Part print with two shaded views. Sizes in mm from the minimum x, y, z corner. A direction names the side the tool comes from. Round coordinates to 2 decimals unless told otherwise and drop trailing zeros. Write each loop counter-clockwise with the first axis right and the second up, starting at its lowest first coordinate (ties: lowest second). Pieces come first, ordered by that corner, then holes. Notation, with made-up numbers: (34, -24.75) -> (72, -24.75) arc R26 cw to (72, 9.25) -> close; hole circle Ø8 at (-4, -1.5). An arc over 180 degrees is marked (long way). Put each result on its own line as item: value. Start each with the question number.
1. Saw through at A-A on y = 8.5. List the corners of the cut face in (x, z) (1 decimal).
2. 3-axis set-ups, long thin cutter, end or side, ignore diameter. For the marked faces 1 and 2: which of +Z, -Z, +X, -X, +Y, -Y reach the whole face in a straight line?
3. Flat gauge pins, fed straight in: P1, Ø2, axis at x = 29, y = 8.5, coming from the +Z side; P2, Ø12, axis at x = 14, z = 8.5, coming from the -Y side; P3, Ø1.9, axis at y = 10, z = 15.5, coming from the +X side. Where does each tip first touch, or does it go through?
4. Saw through at B-B on z = 7.5. List the corners of the cut face in (x, y).
5. Drill centre lines: line 1 (Z direction, x = 5.08, y = 9.75) (1 decimal); line 2 (X direction, y = 8, z = 17.78) (1 decimal); line 3 (Y direction, x = 2.5, z = 21.5). Where is each one in solid material? Low to high. Write a range as from..to.
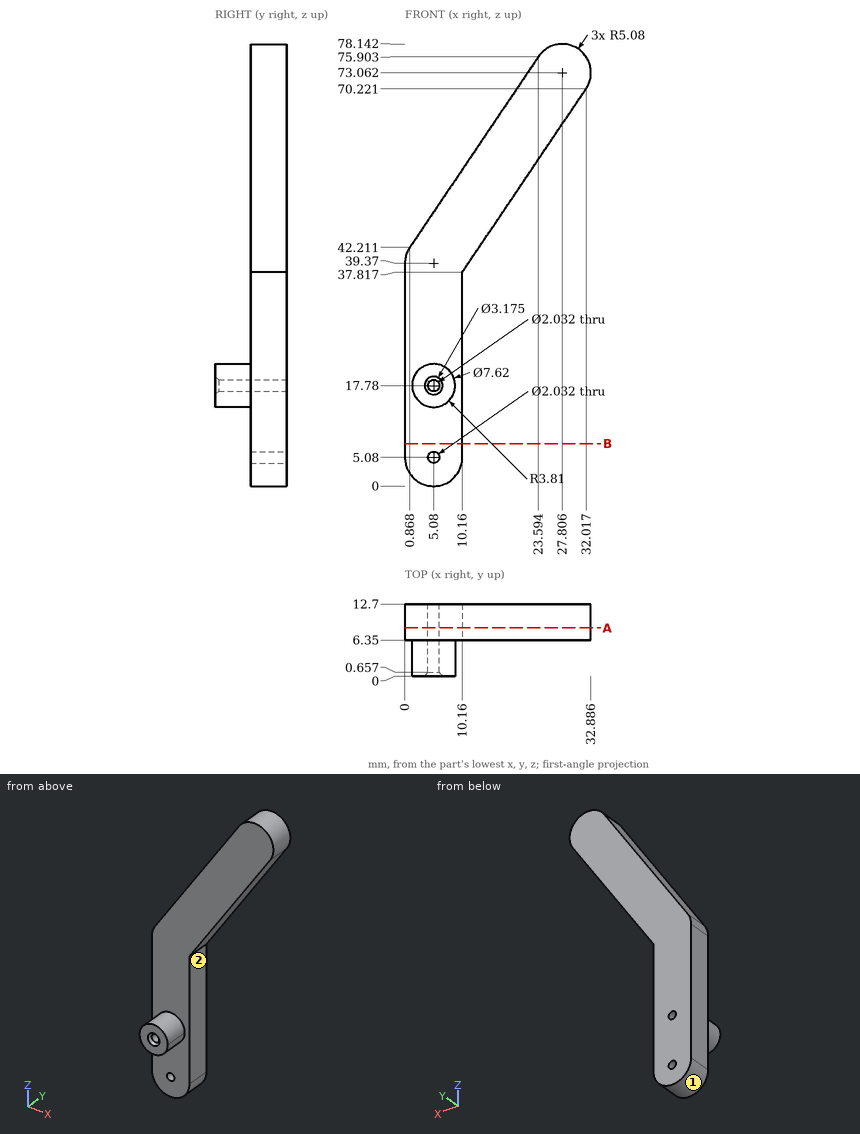
Return value:
1. outline: (0, 5.1) arc R5.1 ccw to (10.2, 5.1) -> (10.2, 37.8) -> (32, 70.2) arc R5.1 ccw to (23.6, 75.9) -> (0.9, 42.2) arc R5.1 ccw to (0, 39.4) -> close; hole circle Ø2 at (5.1, 5.1); hole circle Ø2 at (5.1, 17.8)
2. face 1: -Z, +Y, -Y
2. face 2: -Z, +X, +Y, -Y
3. P1: stops at z = 78.14
3. P2: stops at y = 6.35
3. P3: stops at x = 10.16
4. outline: (0, 6.35) -> (10.16, 6.35) -> (10.16, 12.7) -> (0, 12.7) -> close
5. line 1: z = 0..4.1, 6.1..16.8, 18.8..48.5
5. line 2: x = 0..4.1, 6.1..10.2
5. line 3: y = 6.35..12.7
